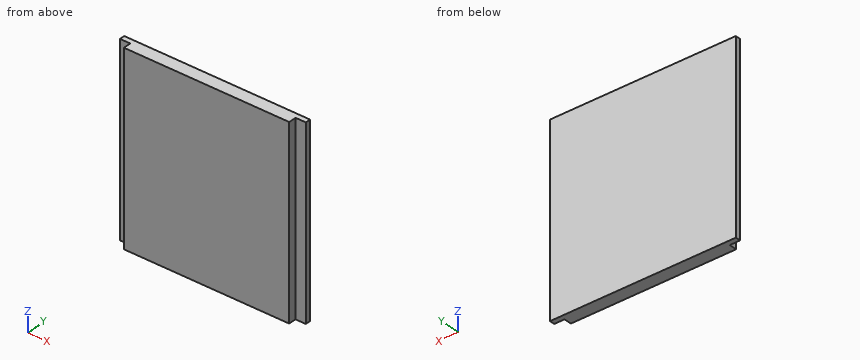
from build123d import *

# Parameters (mm, degrees)
SKETCH017_W               = 32
SKETCH017_H               = 36
EXTRUDE015_DEPTH          = 1.5
SKETCH016_W               = 36
SKETCH016_H               = 36
EXTRUDE014_DEPTH          = 1
FUSION009_PLACEMENT_ANGLE = 90


with BuildPart() as extrude015:
    # Sketch017 (on Face6 of Extrude014) → Extrude015 (new body)
    with BuildSketch(Plane.XY.offset(1)):
        Rectangle(SKETCH017_W, SKETCH017_H)
    extrude(amount=EXTRUDE015_DEPTH)


with BuildPart() as fusion009:
    # Sketch016 → Extrude014 (new body)
    with BuildSketch(Plane.XY):
        Rectangle(SKETCH016_W, SKETCH016_H)
    extrude(amount=EXTRUDE014_DEPTH)

    # Fusion009: union Extrude015
    add(extrude015.part)


with BuildPart() as fusion009_1:
    # Fusion009 placement: moved
    add(fusion009.part.moved(Location((0, -17.5, 0))).rotate(Axis((0, -17.5, 0), (1, 0, 0)), FUSION009_PLACEMENT_ANGLE))


solid = fusion009_1.part
Read the model definition and answer for the solid it produces. Units are mm, in the model's axes. Coordinates: 2 decimals unless noted, no trailing zeros. Loops run counter-clockwise (first coordinate to the right, second up) from the corner with the lowest first, then second, coordinate; pieces in that order, holes last.
Q1. The part is cut by section B-B on y = -19.55. Write down the section's boundary in (x, z).
Q2. Consider probe 1 along X at (y, z) = (-19.5, 3.5); probe 2 along Y at (x, z) = (16.5, -13). Determine where each line is inside the solid, lowest interval first.
Q3. The part is cut by section A-A on z = 13. Write down the section's boundary in (x, y), and give its area (3 significant figures).
Q4. Each of these flat-tipped pins is pushed along its axis until it touches: pin 1 Ø2 at (x, z) = (-17.5, 2.5) entering from -Y; pin 2 Ø0.8 at (y, z) = (-19.5, 6.5) entering from +X. Where does it stop, or does it pass through?
Results below:
1. outline: (-16, -18) - (16, -18) - (16, 18) - (-16, 18) - close
2. probe 1: x = -16 to 16
2. probe 2: y = -18.5 to -17.5
3. outline: (-18, -18.5) - (-16, -18.5) - (-16, -20) - (16, -20) - (16, -18.5) - (18, -18.5) - (18, -17.5) - (-18, -17.5) - close
3. area: 84.0 mm2
4. pin 1: stops at y = -18.5
4. pin 2: stops at x = 16
